Autodesk Inventor part; units mm, degrees
ref_plane "YZ Plane" through (0, 0, 0) normal (1, 0, 0) x (0, 1, 0)
ref_plane "XZ Plane" through (0, 0, 0) normal (0, 1, 0) x (-1, 0, 0)
ref_plane "XY Plane" through (0, 0, 0) normal (0, 0, 1) x (1, 0, 0)
sketch "Sketch1" plane through (0, 0, 0) normal (0, 0, 1) x (1, 0, 0)
  line L0 (0, 0) -> (0, 60)
  line L1 (15, 80) -> (15, 30)
  line L2 (15, 30) -> (90, 30)
  line L3 (90, 30) -> (90, 0)
  line L4 (90, 0) -> (0, 0)
  arc A0 (15, 80) -> (0, 60) centre (19.99, 60.6325) ccw
  dimension "d0" = 60
  dimension "d1" = 90
  dimension "d2" = 30
  dimension "d3" = 75
  dimension "d4" = 50
  dimension "d5" = 20
extrude "Extrusion1" add sketch "Sketch1" along normal mid plane 50
sketch "Sketch2" plane through (90, 0, 25) normal (1, 0, 0) x (0, 0, -1)
  line L0 (50, 30) -> (0, 30)
  arc A0 (40, 45) -> (10, 45) centre (25, 45) ccw
  line L1 (50, 0) -> (0, 0)
  line L2 (50, 80) -> (50, 30)
  line L3 (10, 45) -> (10, 30)
  line L4 (40, 45) -> (40, 30)
  circle A1 centre (25, 45) radius 7.5
  point P0 (25, 0)
  dimension "d10" = 45
  dimension "d11" = 25
  dimension "d13" = 15
  dimension "d14" = 15
extrude "Extrusion2" add sketch "Sketch2" against normal blind 15
sketch "Sketch3" plane through (0, 0, 25) normal (0, 0, 1) x (1, 0, 0)
  point P0 (0, 0)
sketch "Sketch5" plane through (0, 0, 25) normal (0, -1, 0) x (1, 0, 0)
  line L0 (90, 0) -> (15, 0)
  line L1 (0, 0) -> (90, 0)
  circle A0 centre (15, 0) radius 15
  circle A1 centre (75, 0) radius 15
  point P0 (0, -25)
  point P1 (60, 0)
  point P2 (30, 0)
  dimension "d18" = 30
extrude "Extrusion3" add sketch "Sketch5" against normal blind 10 contours L0 L1 A0 | L0 A1 picked at (5.1453, 1.1966) picked at (70.6847, 5.6392)
full round fillet "Full Round Fillet2" first side at (70, 10, 31.6312) centre faces at (60.1942, 3.3333, 27.4062) second side at (50, 0, -8.3333)
sketch "Sketch7" plane through (0, 0, -25) normal (0, -1, 0) x (1, 0, 0)
  line L0 (15, 0) -> (90, 0)
  line L1 (90, 0) -> (0, 0)
  circle A0 centre (15, 0) radius 15
  circle A1 centre (75, 0) radius 15
  line L2 (0, 0) -> (0, 50)
  line L3 (90, 0) -> (90, 50)
  point P0 (0, 25)
  point P1 (30, 0)
  point P2 (60, 0)
  dimension "d21" = 30
  dimension "d22" = 30
extrude "Extrusion4" add sketch "Sketch7" against normal blind 10 contours L0 A0 L1 | L0 A1 picked at (24.8547, -1.1966) picked at (78.2678, -7.6351)
full round fillet "Full Round Fillet4" first side at (18.8878, 10, -29.5122) centre faces at (29.9514, 6.6667, -26.207) second side at (51.6666, 0, 8.3333)
fillet "Fillet1" radius 5 1 edges at (15, 10, 40)
fillet "Fillet2" radius 5 2 edges at (75, 10, -40) (75, 0, -40)
properties part number "Lab 1B A"
Design review of the part built by this model. Coordinates are the model's own, in mm. A direction names the side the tool comes from. Coordinates: 2 decimals unless noted, no trailing zeros. Write each loop counter-clockwise with the first axis right and the second up, starting at its lowest first coordinate (ties: lowest second). Pieces come first, ordered by that corner, then holes. Notation, with made-up numbers: M 71,72 L 127,72 A19 ccw 127,97 Z; hole C -35.5,15.25 d8. An arc over 180 degrees is marked long. Answer as a JSON object with one key per item and string values.
Item 1: Wall thickness on probe 1 along Y at (x, z) = (83, 0); probe 2 along X at (y, z) = (60, -23); probe 3 along Y at (x, z) = (86, 0): over which ranges is each line inside the solid? List them lowest first.
Outcome:
{"probe 1": "0 to 37.5, 52.5 to 60", "probe 2": "0 to 15", "probe 3": "0.1 to 37.5, 52.5 to 60"}
Item 2: Draft analysis for pull direction X (two halves, no side actions). For faces 1 (the flat face through (0, 32, 0)), 2 (the flat face through (52, 30, 0)), 3 (the flat face through (90, 27, 0)), state which applies: pulls with the +X half, pulls with the -X half, needs draft (parallel to the pull), parting line crosses it, or undercut.
Outcome:
{"face 1": "pulls with the -X half", "face 2": "undercut", "face 3": "pulls with the +X half"}
Item 3: Add section C-C, the plane z = -20. Give the boundary of the cut face in (x, y), and give its area (3 significant figures).
Outcome:
{"outline": "M 0,5 A5 ccw 5,0 L 85,0 A5 ccw 90,5 L 90,30 L 15,30 L 15,80 A20 ccw 0,60 Z", "area": "3,360 mm²"}
Item 4: Add section B-B, the plane y = 55.5. Give the boundary of the cut face in (x, z), and give its area (3 significant figures).
Outcome:
{"outline": "M 0,-25 L 15,-25 L 15,25 L 0,25 Z; M 75,-10.71 L 90,-10.71 L 90,10.71 L 75,10.71 Z", "area": "1,070 mm²"}
Item 5: Insertion check: pin 1 Ø15 at (y, z) = (30, -4.5) entering from -X; pin 2 Ø2 at (x, z) = (26, 22.5) entering from +Y; pin 3 Ø12 at (x, y) = (53, 23.5) entering from -Z. Each pin has a flat end and moves straight along its axis. Give the tip position at first contact, or say it passes through.
Outcome:
{"pin 1": "x = 0", "pin 2": "y = 30", "pin 3": "z = -25"}
Item 6: Add section D-D, the plane x = 50. Give the boundary of the cut face in (y, z), and give its area (3 significant figures).
Outcome:
{"outline": "M 0,-25 L 30,-25 L 30,25 L 0,25 Z", "area": "1,500 mm²"}
Item 7: Machinability: for faces 4 (the cylindrical face through (83, 60, 0)), 5 (the cylindrical face through (82.6, 37.68, 1.63)), 6 (the flat face through (15, 10, -29)), which of the approach directions +Z, -Z, +X, -X, +Y, -Y give a long, thin tool a straight path to every point of the face, cutting with its end or side? Answer none if there is none.
Outcome:
{"face 4": "+X, +Y", "face 5": "+X", "face 6": "-Z, +X, -X, +Y"}
Item 8: Add section A-A, the plane z = 0. Give the boundary of the cut face in (x, y), and give its area (3 significant figures).
Outcome:
{"outline": "M 0,5 A5 ccw 5,0 L 85,0 A5 ccw 90,5 L 90,37.5 L 75,37.5 L 75,30 L 15,30 L 15,80 A20 ccw 0,60 Z; M 75,52.5 L 90,52.5 L 90,60 L 75,60 Z", "area": "3,590 mm²"}
